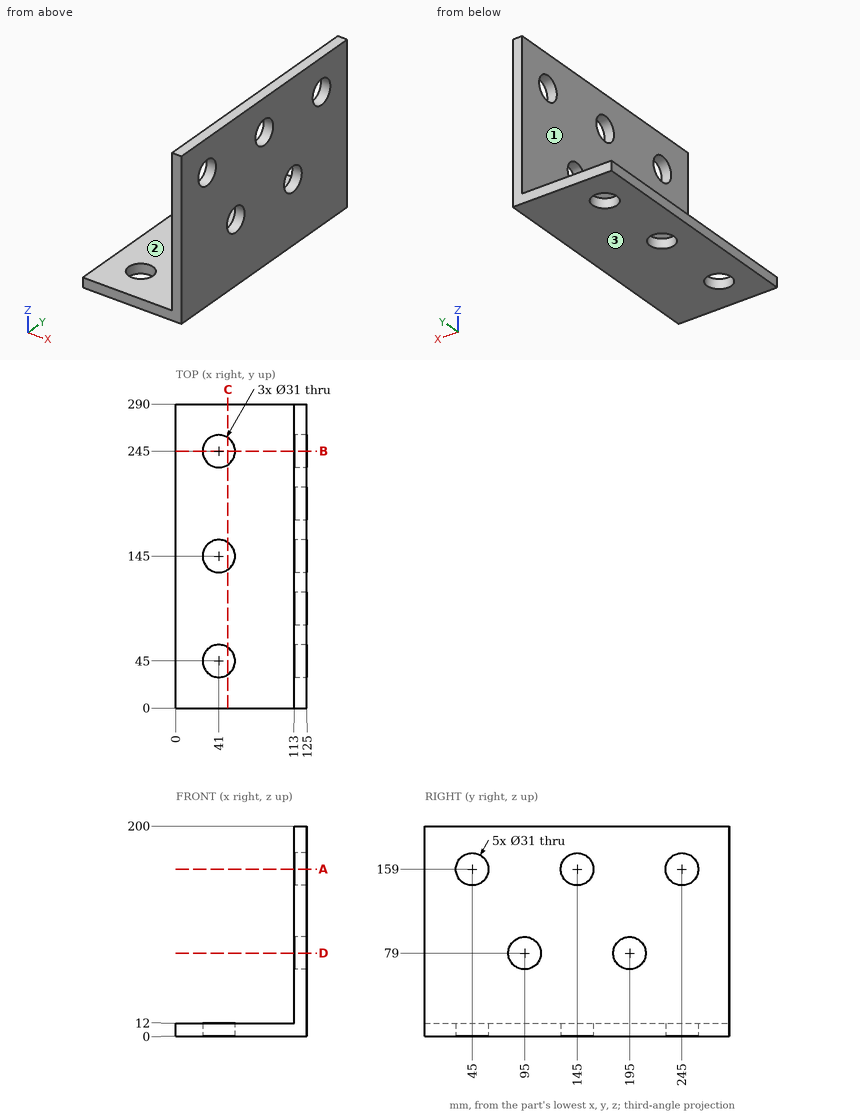
Here's the drawing with two shaded views (mm, measured from the low corner). I have some questions. Coordinates: 2 decimals unless noted, no trailing zeros. Write each loop counter-clockwise with the first axis right and the second up, starting at its lowest first coordinate (ties: lowest second). Pieces come first, ordered by that corner, then holes. Notation, with made-up numbers: (16, 28) - (48, 28) arc R7 cw to (48, 32) - close; hole circle Ø7 at (84.5, -30). An arc over 180 degrees is marked (long way). Return JSON: item names as keys, results as strings.
Q1. If we section it at D-D (z = 79): Please give me the cut outline in (x, y), then the cut area to 3 significant figures.
Computed values:
{"outline": "(113, 0) - (125, 0) - (125, 79.5) - (113, 79.5) - close; (113, 110.5) - (125, 110.5) - (125, 179.5) - (113, 179.5) - close; (113, 210.5) - (125, 210.5) - (125, 290) - (113, 290) - close", "area": "2,740 mm2"}
Q2. I'm going to push a flat-ended pin straight in: pin 1 Ø1.5 at (x, y) = (46, 78.5) entering from +Z. Where does the tip first touch, or does it pass through?
Computed values:
{"pin 1": "stops at z = 12"}
Q3. If we section it at A-A (z = 159): Please give me the cut outline in (x, y), then the cut area to 3 significant figures.
Computed values:
{"outline": "(113, 0) - (125, 0) - (125, 29.5) - (113, 29.5) - close; (113, 60.5) - (125, 60.5) - (125, 129.5) - (113, 129.5) - close; (113, 160.5) - (125, 160.5) - (125, 229.5) - (113, 229.5) - close; (113, 260.5) - (125, 260.5) - (125, 290) - (113, 290) - close", "area": "2,360 mm2"}
Q4. If we section it at B-B (y = 245): Please give me the cut outline in (x, z), then the cut area to 3 significant figures.
Computed values:
{"outline": "(0, 0) - (25.5, 0) - (25.5, 12) - (0, 12) - close; (56.5, 0) - (125, 0) - (125, 143.5) - (113, 143.5) - (113, 12) - (56.5, 12) - close; (113, 174.5) - (125, 174.5) - (125, 200) - (113, 200) - close", "area": "3,010 mm2"}
Q5. Please list where these lines run through material, in increasing order: L1, parallel to Y at x = 41, z = 9; L2, parallel to Y at x = 113.5, z = 148.5; L3, parallel to X at y = 196, z = 98. Write a range as from..to.
Computed values:
{"L1": "y = 0..29.5, 60.5..129.5, 160.5..229.5, 260.5..290", "L2": "y = 0..33.6, 56.4..133.6, 156.4..233.6, 256.4..290", "L3": "x = 113..125"}
Q6. If we section it at C-C (x = 49.5): Please give me the cut outline in (y, z), then the cut area to 3 significant figures.
Computed values:
{"outline": "(0, 0) - (32.04, 0) - (32.04, 12) - (0, 12) - close; (57.96, 0) - (132.04, 0) - (132.04, 12) - (57.96, 12) - close; (157.96, 0) - (232.04, 0) - (232.04, 12) - (157.96, 12) - close; (257.96, 0) - (290, 0) - (290, 12) - (257.96, 12) - close", "area": "2,550 mm2"}
Q7. Thinking about a two-plate mould opening in Z: for the marked faces 1, 2 and 3, which applies, +Z half, -Z half, draft (parallel to the pull), parting line (faces both ways), or undercut?
Computed values:
{"face 1": "draft", "face 2": "+Z half", "face 3": "-Z half"}
